The model under review builds one solid part; all positions refer to its coordinate system, in mm. Face numbers are marked on the shaded views. A direction names the side the tool comes from. Round coordinates to 2 decimals unless told otherwise and drop trailing zeros. Order: outer loops, then holes, each group sorted by start corner. A loop starts at its lowest first (then second) coordinate and runs counter-clockwise, first axis right, second up. Notation, with made-up numbers: (-26, -32) -> (20, -32) arc R32 ccw to (20, -4) -> close; hole circle Ø9 at (62.5, 89.25). An arc over 180 degrees is marked (long way). Use a Markdown table: item, result. Add a question column.
```python
from build123d import *

# Parameters (mm, degrees)
BOSS_EXTRUDE1_DEPTH     = 50
SKETCH2_W               = 190
SKETCH2_H               = 100
BOSS_EXTRUDE2_DEPTH     = 5
SKETCH3_W               = 190
SKETCH3_H               = 50
BOSS_EXTRUDE3_DEPTH     = 5
CUT_EXTRUDE1_DEPTH      = 291
CUT_EXTRUDE1_DEPTH_BACK = 20
SKETCH4_R               = 5
CUT_EXTRUDE2_DEPTH      = 291
CUT_EXTRUDE2_DEPTH_BACK = 21
SKETCH5_R               = 5


with BuildPart() as part:
    # Sketch1 → Boss-Extrude1 (new body)
    with BuildSketch(Plane(origin=(0, 0, 0), x_dir=(1, 0, 0), z_dir=(0, 1, 0))):
        Polygon((-68.351724138, 159.884429765), (-68.351724138, 219.884429765), (-38.351724138, 219.884429765), (-38.351724138, 224.884429765), (-118.351724138, 224.884429765), (-118.351724138, 219.884429765), (-88.351724138, 219.884429765), (-88.351724138, 159.884429765), (-168.351724138, 159.884429765), (-168.351724138, 187.384429765), (-173.351724138, 187.384429765), (-173.351724138, 154.884429765), (-88.351724138, 154.884429765), (-88.351724138, -125.115570235), (-173.351724138, -125.115570235), (-173.351724138, -157.665570235), (-168.351724138, -157.665570235), (-168.351724138, -130.115570235), (-88.351724138, -130.115570235), (-88.351724138, -190.115570235), (-118.351724138, -190.115570235), (-118.351724138, -195.115570235), (-38.351724138, -195.115570235), (-38.351724138, -190.115570235), (-68.351724138, -190.115570235), (-68.351724138, -130.115570235), (11.648275862, -130.115570235), (11.648275862, -157.615570235), (16.648275862, -157.615570235), (16.648275862, -125.115570235), (-68.351724138, -125.115570235), (-68.351724138, 154.884429765), (16.648275862, 154.884429765), (16.648275862, 187.384429765), (11.648275862, 187.384429765), (11.648275862, 159.884429765), align=None)
    extrude(amount=BOSS_EXTRUDE1_DEPTH)

    # Sketch2 → Boss-Extrude2 (add)
    with BuildSketch(Plane(origin=(0, 0, -224.884429765), x_dir=(-1, 0, 0), z_dir=(0, 0, -1))):
        with Locations((78.351724138, 25)):
            Rectangle(SKETCH2_W, SKETCH2_H)
    extrude(amount=-BOSS_EXTRUDE2_DEPTH)

    # Sketch3 → Boss-Extrude3 (add)
    with BuildSketch(Plane.XY.offset(195.115570235)):
        with Locations((-78.351724138, 25)):
            Rectangle(SKETCH3_W, SKETCH3_H)
    extrude(amount=-BOSS_EXTRUDE3_DEPTH)

    # Sketch4 → Cut-Extrude1 (cut, two sides: drawn at the far end of the back side and taken through both)
    with BuildSketch(Plane(origin=(0, 0, 125.115570235), x_dir=(-1, 0, 0), z_dir=(0, 0, -1)).offset(-CUT_EXTRUDE1_DEPTH_BACK)):
        with Locations((155.851724138, 25)):
            Circle(SKETCH4_R)
    extrude(amount=CUT_EXTRUDE1_DEPTH + CUT_EXTRUDE1_DEPTH_BACK, mode=Mode.SUBTRACT)

    # Sketch5 → Cut-Extrude2 (cut, two sides: drawn at the far end of the back side and taken through both)
    with BuildSketch(Plane(origin=(0, 0, 125.115570235), x_dir=(-1, 0, 0), z_dir=(0, 0, -1)).offset(-CUT_EXTRUDE2_DEPTH_BACK)):
        with Locations(Location((0.851724138, 25, 0), (0, 0, 180))):
            Circle(SKETCH5_R)
    extrude(amount=CUT_EXTRUDE2_DEPTH + CUT_EXTRUDE2_DEPTH_BACK, mode=Mode.SUBTRACT)


solid = part.part
```
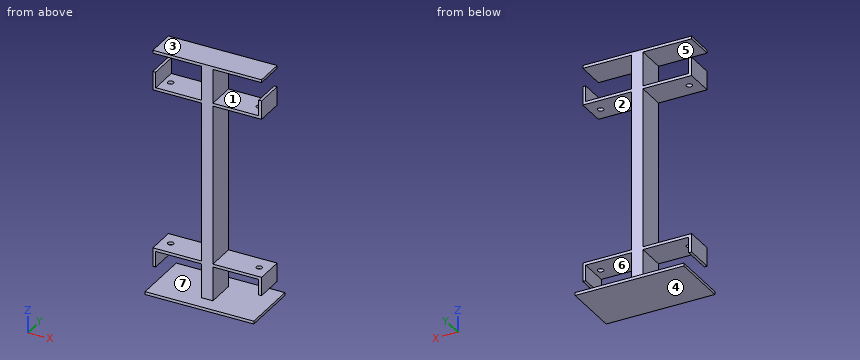
Q1. Mouldability with a two-part tool opening along X and no side actions: class the marked faces 6 and 7 as pulls with the +X half, pulls with the -X half, needs draft (parallel to the pull), parting line crosses it, or undercut.
Q2. Insertion check: pin 1 (3 mm diameter, centred on y = 6.5, z = -14, fed in from -X); pin 2 (1.5 mm diameter, centred on y = 6.5, z = -32, fed in from +X); pin 3 (12 mm diameter, centred on x = -8.5, z = 129, fed in from +Y). Each pin has a flat end and moves straight along its axis. Give the tip position at first contact, or say it passes through.
Q3. Add section A-A (x = -118.5). Write out the cut boundary in (y, z), then the cut area to 3 significant figures.
Q4. Add section C-C (y = 25). State how many separate pieces and enclosed holes the cut face has, then the cut area to 3 significant figures.
Q5. Add section B-B (x = -0.5). Write out the cut boundary in (y, z).
Q6. Wall thickness on line 1 (Z direction, x = -26, y = 6); line 2 (Z direction, x = -41.5, y = -11); line 3 (X direction, y = 40.5, z = -193.5): over which ranges is each line inside the solid? List them lowest first. Write a range as [from, to].
Q7. Add section D-D (z = -48). Write out the cut boundary in (x, y).
Q8. Machinability: for the marked faces 1, 2, 3, 4 and 5, which of the approach directions +Z, -Z, +X, -X, +Y, -Y give a long, thin tool a straight path to every point of the face, cutting with its end or side? Answer none if there is none.
Report:
| question | item | result |
|---|---|---|
| 1 | face 6 | undercut |
| 1 | face 7 | needs draft |
| 2 | pin 1 | stops at x = -88.35 |
| 2 | pin 2 | stops at x = -68.35 |
| 2 | pin 3 | stops at y = 50 |
| 3 | outline | (-25, -224.88) -> (75, -224.88) -> (75, -219.88) -> (-25, -219.88) -> close; (0, -159.88) -> (50, -159.88) -> (50, -154.88) -> (0, -154.88) -> close; (0, 125.12) -> (50, 125.12) -> (50, 130.12) -> (0, 130.12) -> close; (0, 190.12) -> (50, 190.12) -> (50, 195.12) -> (0, 195.12) -> close |
| 3 | area | 1,250 mm² |
| 4 | separate pieces | 5 |
| 4 | enclosed holes | 0 |
| 4 | area | 12,200 mm² |
| 5 | outline | (-25, -224.88) -> (75, -224.88) -> (75, -219.88) -> (-25, -219.88) -> close; (0, -159.88) -> (20.01, -159.88) -> (20.01, -154.88) -> (0, -154.88) -> close; (0, 125.12) -> (20.01, 125.12) -> (20.01, 130.12) -> (0, 130.12) -> close; (0, 190.12) -> (50, 190.12) -> (50, 195.12) -> (0, 195.12) -> close; (29.99, -159.88) -> (50, -159.88) -> (50, -154.88) -> (29.99, -154.88) -> close; (29.99, 125.12) -> (50, 125.12) -> (50, 130.12) -> (29.99, 130.12) -> close |
| 6 | line 1 | z = [-224.88, -219.88], [-159.88, -154.88], [125.12, 130.12], [190.12, 195.12] |
| 6 | line 2 | z = [-224.88, -219.88] |
| 6 | line 3 | x = [-88.35, -68.35] |
| 7 | outline | (-88.35, 0) -> (-68.35, 0) -> (-68.35, 50) -> (-88.35, 50) -> close |
| 8 | face 1 | +Y, -Y |
| 8 | face 2 | +X, +Y, -Y |
| 8 | face 3 | +Z, +X, -X, +Y, -Y |
| 8 | face 4 | -Z, +X, -X, +Y, -Y |
| 8 | face 5 | -X, +Y, -Y |
